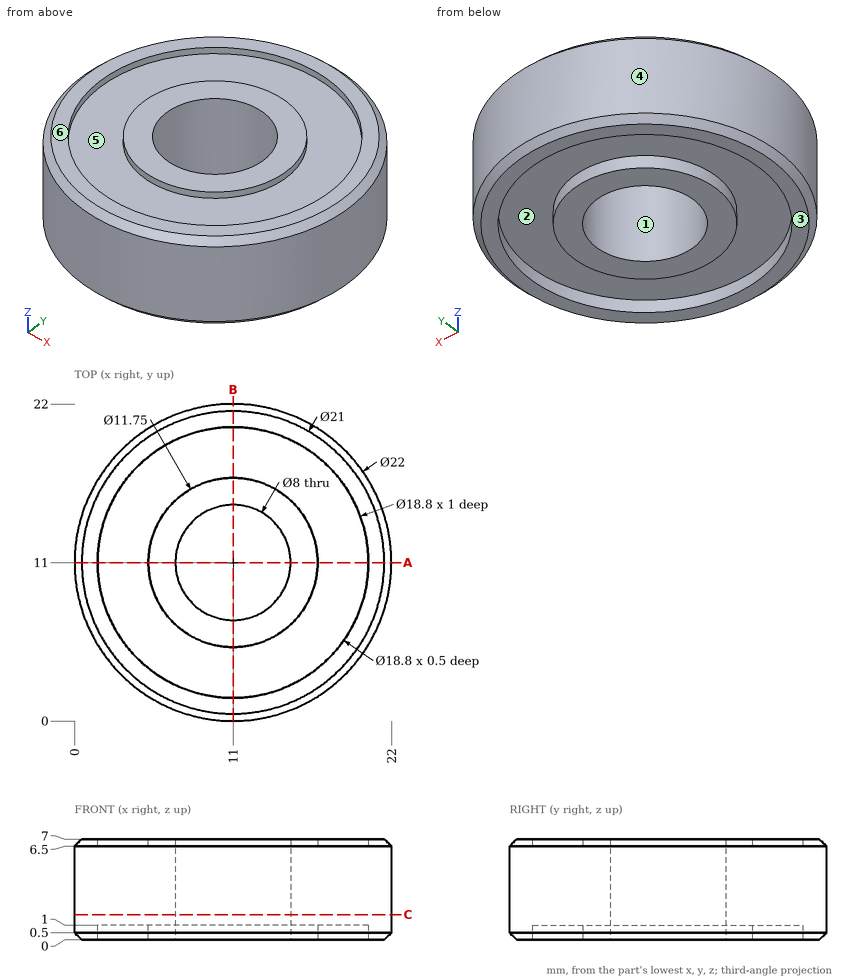
Answer from the drawing. Dimensions are ordinates in mm from the lowest x, y and z of the part. A direction names the side the tool comes from. Give positions to 0.01 mm unless a question says otherwise; leave off trailing zeros. Write each loop counter-clockwise with the first axis right and the second up, starting at its lowest first coordinate (ties: lowest second). Pieces come first, ordered by that corner, then holes. Notation, with made-up numbers: (20, 32.25) -> (47, 32.25) arc R16 ccw to (47, 58.25) -> close; hole circle Ø10 at (32, 31). An arc over 180 degrees is marked (long way). One line per question, with ' | ' between items. Start each with the question number.
1. Section C-C (z = 1.75) is taken. Determine the outline of the cut face in (x, y).
2. For the marked faces 5 and 6, determine the directions among +Z, -Z, +X, -X, +Y, -Y from which every point of the face is accessible in a straight line to the end or side of a thin tool.
3. For a pull along X with two mould halves and no side action, classify the marked faces 1, 2, 3 and 4 as pulls with the +X half, pulls with the -X half, needs draft (parallel to the pull), parting line crosses it, or undercut.
4. Given pin 1 Ø3 at (y, z) = (17.5, 4.5) entering from +X; pin 2 Ø1 at (x, z) = (12.5, 6) entering from +Y; pin 3 Ø10.5 at (x, y) = (11, 11) entering from -Z; pin 4 Ø4 at (x, z) = (2, 1.5) entering from +Y, each flat-ended and moving along its own axis, determine where each tip first touches the part or whether it passes through.
5. Find the intervals of material crossed by probe 1 along Y at (x, z) = (11, 0.4) (3 decimals); probe 2 along Z at (x, y) = (11, 2); probe 3 along Y at (x, z) = (11, 4), in increasing order.
6. Section A-A (y = 11) is taken. Determine the outline of the cut face in (x, z) (3 decimals), plus the area to 3 significant figures.
Response values:
1) outline: circle Ø22 at (11, 11); hole circle Ø8 at (11, 11)
2) face 5: +Z | face 6: +Z, +X, -X, +Y, -Y
3) face 1: undercut | face 2: undercut | face 3: needs draft | face 4: parting line crosses it
4) pin 1: x = 20.8 | pin 2: y = 21.95 | pin 3: z = 0 | pin 4: y = 19.49
5) probe 1: 0.1 to 1.6, 5.125 to 7, 15 to 16.875, 20.4 to 21.9 | probe 2: 1 to 6.5 | probe 3: 0 to 7, 15 to 22
6) outline: (0, 0.5) -> (0.5, 0) -> (1.6, 0) -> (1.6, 1) -> (5.125, 1) -> (5.125, 0) -> (7, 0) -> (7, 7) -> (5.125, 7) -> (5.125, 6.5) -> (1.6, 6.5) -> (1.6, 7) -> (0.5, 7) -> (0, 6.5) -> close; (15, 0) -> (16.875, 0) -> (16.875, 1) -> (20.4, 1) -> (20.4, 0) -> (21.5, 0) -> (22, 0.5) -> (22, 6.5) -> (21.5, 7) -> (20.4, 7) -> (20.4, 6.5) -> (16.875, 6.5) -> (16.875, 7) -> (15, 7) -> close | area: 86.9 mm2
